For this review, take the finished solid that the model builds, in its own axes (mm). A direction names the side the tool comes from. Coordinates: 2 decimals unless noted, no trailing zeros. Loops run counter-clockwise (first coordinate to the right, second up) from the corner with the lowest first, then second, coordinate; pieces in that order, holes last. Notation, with made-up numbers: M -15,45.25 L 43,45.25 A37 ccw 43,83.25 Z; hole C -25.5,45.25 d7. An arc over 180 degrees is marked long. Write item = value, one per line.
from build123d import *

# Parameters (mm, degrees)
SKETCH_1_W          = 21
SKETCH_1_H          = 38
SKETCH_1_W_2        = 15
SKETCH_1_H_2        = 32
EXTRUDE_1_DEPTH     = 18
SKETCH_2_W          = 21
SKETCH_2_H          = 38
EXTRUDE_2_DEPTH     = 3
SKETCH_3_W          = 15
SKETCH_3_H          = 15
CUT_EXTRUDE_1_DEPTH = 3


with BuildPart() as part:
    # 草圖1 → 填料-伸長1 (new body)
    with BuildSketch(Plane.XY):
        with Locations((-0.498060931, -7.683431953)):
            Rectangle(SKETCH_1_W, SKETCH_1_H)
        with Locations((-0.498060931, -7.683431953)):
            Rectangle(SKETCH_1_W_2, SKETCH_1_H_2, mode=Mode.SUBTRACT)
    extrude(amount=EXTRUDE_1_DEPTH)

    # 草圖2 → 填料-伸長2 (add)
    with BuildSketch(Plane(origin=(0, 0, 0), x_dir=(-1, 0, 0), z_dir=(0, 0, -1))):
        with Locations((0.498060931, -7.683431953)):
            Rectangle(SKETCH_2_W, SKETCH_2_H)
    extrude(amount=EXTRUDE_2_DEPTH)

    # 草圖3 → 除料-伸長1 (cut)
    with BuildSketch(Plane.XZ.offset(26.683431953)):
        with Locations((-0.498060931, 10.5)):
            Rectangle(SKETCH_3_W, SKETCH_3_H)
    extrude(amount=-CUT_EXTRUDE_1_DEPTH, mode=Mode.SUBTRACT)


solid = part.part
Q1. Add section A-A (z = 1.5). Write out the cut boundary in (x, y), and give its area (3 significant figures).
Solved:
outline = M -11,-26.68 L 10,-26.68 L 10,11.32 L -11,11.32 Z; hole M -8,-23.68 L 7,-23.68 L 7,8.32 L -8,8.32 Z
area = 318 mm²
Q2. For line 1 along X through (y, z) = (-22, 5.75); line 2 along Y through (x, z) = (0.25, 0.25); line 3 along Z through (x, y) = (3, -11.5), list the stretches that pass through material, from the lowest coordinate up.
Solved:
line_1 = -11 to -8, 7 to 10
line_2 = -26.68 to -23.68, 8.32 to 11.32
line_3 = -3 to 0
Q3. For pin 1 Ø6 at (x, z) = (2, 7) entering from -Y; pin 2 Ø1.5 at (x, y) = (1, -25.5) entering from +Z, all flat-tipped, find the tip position at first contact; note any pin that passes through.
Solved:
pin_1 = 8.32
pin_2 = 3
Q4. Machinability: for faces 1 (the face through (0, -26.683, 1)), 2 (the face through (-7.998, -9, 9)), which of the approach directions +Z, -Z, +X, -X, +Y, -Y give a long, thin tool a straight path to every point of the face, cutting with its end or side? Answer none if there is none.
Solved:
face_1 = +Z, -Z, +X, -X, -Y
face_2 = +Z
Q5. Add section C-C (z = 9.5). Write out the cut boundary in (x, y), and give its area (3 significant figures).
Solved:
outline = M -11,-26.68 L -8,-26.68 L -8,8.32 L 7,8.32 L 7,-26.68 L 10,-26.68 L 10,11.32 L -11,11.32 Z
area = 273 mm²
Q6. Draft analysis for pull direction Y (two halves, no side actions). For faces 3 (the face through (0, 11.317, 8)), 4 (the face through (-1, 8.317, 9)), 5 (the face through (0, -7, 0)), 6 (the face through (-1, -25, 3)), state which applies: +Y half, -Y half, draft (parallel to the pull), parting line (faces both ways), or undercut.
Solved:
face_3 = +Y half
face_4 = undercut
face_5 = undercut
face_6 = draft
Q7. Add section B-B (x = -0.75). Write out the cut boundary in (y, z), and give its area (3 significant figures).
Solved:
outline = M -26.68,-3 L 11.32,-3 L 11.32,18 L 8.32,18 L 8.32,0 L -23.68,0 L -23.68,3 L -26.68,3 Z
area = 177 mm²
